from build123d import *

# Parameters (mm, degrees)
BOSS_EXTRUDE1_DEPTH = 0.12
SKETCH2_W           = 12.5
SKETCH2_H           = 4
BOSS_EXTRUDE2_DEPTH = 0.18
FILLET1_R           = 1


with BuildPart() as part:
    # Sketch1 → Boss-Extrude1 (new body)
    with BuildSketch(Plane(origin=(0, 0, 0), x_dir=(1, 0, 0), z_dir=(0, 1, 0))):
        Polygon((-4.25, 0), (4.25, 0), (4.25, -8.5), (3, -8.5), (3, -66.5), (6.25, -66.5), (6.25, -70.5), (-6.25, -70.5), (-6.25, -66.5), (-3, -66.5), (-3, -8.5), (-4.25, -8.5), align=None)
    extrude(amount=BOSS_EXTRUDE1_DEPTH)

    # Sketch2 → Boss-Extrude2 (add)
    with BuildSketch(Plane(origin=(0, 0.12, 0), x_dir=(1, 0, 0), z_dir=(0, 1, 0))):
        with Locations((0, -68.5)):
            Rectangle(SKETCH2_W, SKETCH2_H)
    extrude(amount=BOSS_EXTRUDE2_DEPTH)

    # Fillet1
    fillet1_edges = [part.edges().sort_by_distance(p)[0] for p in [
        (3, 0.06, 8.5),
        (3, 0.06, 66.5),
        (6.25, 0.15, 66.5),
        (-6.25, 0.15, 66.5),
        (-3, 0.06, 66.5),
        (-3, 0.06, 8.5),
    ]]
    fillet(fillet1_edges, radius=FILLET1_R)


solid = part.part
The model under review builds one solid part; all positions refer to its coordinate system, in mm. Round coordinates to 2 decimals unless told otherwise and drop trailing zeros. Write each loop counter-clockwise with the first axis right and the second up, starting at its lowest first coordinate (ties: lowest second). Pieces come first, ordered by that corner, then holes. Notation, with made-up numbers: M 76,31 L 113,31 A16 ccw 113,50 Z; hole C 3,70 d8. An arc over 180 degrees is marked long. Use a Markdown table: item, result. Add a question column.
Q1. To check wall thickness, follow line 1 (Z direction, x = -2.5, y = 0.2); line 2 (X direction, y = 0.05, z = 9.5). State the ranges of each line that lie inside material, in increasing order.
Q2. We need section B-B, the plane x = 2. State the section outline as (y, z) points, plus the area to 3 significant figures.
Q3. We need section A-A, the plane y = 0.2. State the section outline as (x, z) points, plus the area to 3 significant figures.
Q4. We need section C-C, the plane z = 6.5. State the section outline as (x, y) points.
Q5. Insertion check: pin 1 (6 mm diameter, centred on x = 1, z = 20.5, fed in from +Y). The pin has a flat end and moves straight along its axis. Give the tip position at first contact, or say it passes through.
Findings below:
| question | item | result |
|---|---|---|
| 1 | line 1 | z = 66.5 to 70.5 |
| 1 | line 2 | x = -3 to 3 |
| 2 | outline | M 0,0 L 0.12,0 L 0.12,66.5 L 0.3,66.5 L 0.3,70.5 L 0,70.5 Z |
| 2 | area | 9.18 mm² |
| 3 | outline | M -6.25,67.5 A1 ccw -5.25,66.5 L 5.25,66.5 A1 ccw 6.25,67.5 L 6.25,70.5 L -6.25,70.5 Z |
| 3 | area | 49.6 mm² |
| 4 | outline | M -4.25,0 L 4.25,0 L 4.25,0.12 L -4.25,0.12 Z |
| 5 | pin 1 | stops at y = 0.12 |
